Read the model definition and answer for the solid it produces. Units are mm, in the model's axes. A direction names the side the tool comes from. Give positions to 0.01 mm unless a question says otherwise; leave off trailing zeros. Order: outer loops, then holes, each group sorted by start corner. A loop starts at its lowest first (then second) coordinate and runs counter-clockwise, first axis right, second up. Notation, with made-up numbers: M 28.5,33 L 58.5,33 A14 cw 58.5,42 Z; hole C -17.75,-31 d10. An arc over 180 degrees is marked long. One line per item, written item: value.
from build123d import *

# Parameters (mm, degrees)
SKETCH1_W           = 70
SKETCH1_H           = 38
SKETCH1_R           = 2.15
BOSS_EXTRUDE1_DEPTH = 14
FILLET1_R           = 4
SKETCH2_R           = 16.5
BOSS_EXTRUDE2_DEPTH = 22.6
BOSS_EXTRUDE3_START = 2.2
SKETCH3_R           = 6.5
BOSS_EXTRUDE3_DEPTH = 2.2
SKETCH4_R           = 6.5
BOSS_EXTRUDE4_DEPTH = 2.2


with BuildPart() as part:
    # Sketch1 → Boss-Extrude1 (new body)
    with BuildSketch(Plane.XY):
        with Locations((35, 19)):
            Rectangle(SKETCH1_W, SKETCH1_H)
        with Locations((24, 35)):
            Circle(SKETCH1_R, mode=Mode.SUBTRACT)
        with Locations((24, 3)):
            Circle(SKETCH1_R, mode=Mode.SUBTRACT)
        with BuildLine():
            Line((13.654248689, 22), (18.945751311, 22))
            ThreePointArc((18.945751311, 22), (16.3, 15), (13.654248689, 22))
        make_face(mode=Mode.SUBTRACT)
    extrude(amount=BOSS_EXTRUDE1_DEPTH)

    # Fillet1
    fillet1_edges = [part.edges().sort_by_distance(p)[0] for p in [
        (0, 38, 7),
        (70, 38, 7),
        (70, 0, 7),
        (0, 0, 7),
    ]]
    fillet(fillet1_edges, radius=FILLET1_R)

    # Sketch2 → Boss-Extrude2 (add)
    with BuildSketch(Plane(origin=(0, 0, 0), x_dir=(-1, 0, 0), z_dir=(0, 0, -1))):
        with Locations((-48.753788749, 19)):
            Circle(SKETCH2_R)
    extrude(amount=BOSS_EXTRUDE2_DEPTH)

    # Sketch3 → Boss-Extrude3 (add)
    with BuildSketch(Plane(origin=(0, 0, 0), x_dir=(-1, 0, 0), z_dir=(0, 0, -1)).offset(BOSS_EXTRUDE3_START)):
        with Locations((-16.3, 19)):
            Circle(SKETCH3_R)
        with BuildLine():
            Line((-18.945751311, 22), (-13.654248689, 22))
            ThreePointArc((-13.654248689, 22), (-16.3, 15), (-18.945751311, 22))
        make_face(mode=Mode.SUBTRACT)
    extrude(amount=-BOSS_EXTRUDE3_DEPTH)

    # Sketch4 → Boss-Extrude4 (add)
    with BuildSketch(Plane.XY.offset(14)):
        with Locations(Location((16.3, 19, 0), (0, 0, 180))):
            Circle(SKETCH4_R)
        with BuildLine():
            Line((13.654248689, 22), (18.945751311, 22))
            ThreePointArc((18.945751311, 22), (16.3, 15), (13.654248689, 22))
        make_face(mode=Mode.SUBTRACT)
    extrude(amount=BOSS_EXTRUDE4_DEPTH)


solid = part.part
1) Find section C-C, the plane y = 23.5. Write down the section's boundary in (x, z), plus the area to 3 significant figures.
Reported:
outline: M 0,0 L 11.61,0 L 11.61,-2.2 L 20.99,-2.2 L 20.99,0 L 32.88,0 L 32.88,-22.6 L 64.63,-22.6 L 64.63,0 L 70,0 L 70,14 L 20.99,14 L 20.99,16.2 L 11.61,16.2 L 11.61,14 L 0,14 Z
area: 1,740 mm^2
2) Consider probe 1 along X at (y, z) = (19, 15.05); probe 2 along Y at (x, z) = (16.3, 15.35); probe 3 along Z at (x, y) = (13, 24.5). Determine where each line is inside the solid, lowest interval first.
Reported:
probe 1: x = 9.8 to 12.3, 20.3 to 22.8
probe 2: y = 12.5 to 15, 22 to 25.5
probe 3: z = -2.2 to 16.2
3) Which of the six approach directions +Z, -Z, +X, -X, +Y, -Y give full straight-line access (tool end or side, diameter ignored) to faces 1 (the face through (0, 19, 7)), 2 (the face through (1.141, 1.203, 7.098)), 3 (the face through (21.091, 14.607, 15.085)), 4 (the face through (41.14, 4.36, -11.14)), 5 (the face through (16.4, 14.8, -2.2))?
Reported:
face 1: +Z, -Z, -X, +Y, -Y
face 2: +Z, -Z, -X, -Y
face 3: +Z
face 4: -Z
face 5: -Z, -X, +Y, -Y
4) Find section A-A, the plane x = 24. Write down the section's boundary in (y, z).
Reported:
outline: M 0,0 L 0.85,0 L 0.85,14 L 0,14 Z; M 5.15,0 L 32.85,0 L 32.85,14 L 5.15,14 Z; M 37.15,0 L 38,0 L 38,14 L 37.15,14 Z
5) Each of these flat-tipped pins is pushed along its axis until it touches: pin 1 Ø4 at (x, y) = (24, 3) entering from +Z; pin 2 Ø2 at (x, z) = (47.5, -8.5) entering from -Y; pin 3 Ø0.7 at (x, z) = (16, -1.5) entering from -Y; pin 4 Ø7 at (x, y) = (16.3, 19) entering from +Z. Where does it stop, or does it pass through?
Reported:
pin 1: passes through
pin 2: stops at y = 2.5
pin 3: stops at y = 12.5
pin 4: stops at z = 16.2
6) Find section D-D, the plane x = 38. Write down the section's boundary in (y, z).
Reported:
outline: M 0,0 L 6.49,0 L 6.49,-22.6 L 31.51,-22.6 L 31.51,0 L 38,0 L 38,14 L 0,14 Z
7) Determine the mould class of faces 6 (the face through (1.141, 36.797, 7.098)), 7 (the face through (49, 19, -22.6)), 8 (the face through (70, 19, 7)), 9 (the face through (17.146, 25.445, -1.115)) for opening direction X: +X half, -X half, draft (parallel to the pull), parting line (faces both ways), or undercut.
Reported:
face 6: -X half
face 7: draft
face 8: +X half
face 9: undercut
8) Find section B-B, the plane z = 2. Write down the section's boundary in (x, y).
Reported:
outline: M 0,4 A4 ccw 4,0 L 66,0 A4 ccw 70,4 L 70,34 A4 ccw 66,38 L 4,38 A4 ccw 0,34 Z; hole M 13.65,22 A4 ccw long 18.95,22 Z; hole C 24,3 d4.3; hole C 24,35 d4.3
